Model file for the job. Use its own axes, mm. Give positions to 0.01 mm unless a question says otherwise; leave off trailing zeros. Loops run counter-clockwise (first coordinate to the right, second up) from the corner with the lowest first, then second, coordinate; pieces in that order, holes last. Notation, with made-up numbers: M -19,89.5 L 20,89.5 A33 ccw 20,126.5 Z; hole C 7,55 d8. An arc over 180 degrees is marked long. Answer in a Markdown table with one row per item.
```python
from build123d import *

# Parameters (mm, degrees)
SKETCH1_R           = 4
BOSS_EXTRUDE1_DEPTH = 6
FILLET1_R           = 6
CUT_EXTRUDE1_DEPTH  = 6
FILLET3_R           = 5
SKETCH3_R           = 5.01
CUT_EXTRUDE2_DEPTH  = 10
SKETCH4_W           = 10
SKETCH4_H           = 5
CUT_EXTRUDE3_DEPTH  = 10


with BuildPart() as part:
    # Sketch1 → Boss-Extrude1 (new body)
    with BuildSketch(Plane(origin=(0, 0, 0), x_dir=(1, 0, 0), z_dir=(0, 1, 0))):
        Polygon((277.331893801, -59.723964411), (274.249458289, -59.723964411), (270.793440906, -59.723964411), (225, 0), (95, 0), (95, -35), (0, -35), (0, -135), (95, -135), (95, -170), (225, -170), (270.793440906, -110.276035589), (274.249458289, -110.276035589), (277.331893801, -110.276035589), (323.076052888, -138.788463278), (323.076052888, -148.788463278), (333.076052888, -148.788463278), (368.076052888, -128.788463278), (368.076052888, -41.211536722), (333.076052888, -21.211536722), (323.076052888, -21.211536722), (323.076052888, -31.211536722), align=None)
        with Locations(Location((333.076052888, -138.788463278, 0), (0, 0, 270))):
            Circle(SKETCH1_R, mode=Mode.SUBTRACT)
        with Locations(Location((333.076052888, -31.211536722, 0), (0, 0, 90))):
            Circle(SKETCH1_R, mode=Mode.SUBTRACT)
    extrude(amount=BOSS_EXTRUDE1_DEPTH)

    # Fillet1
    fillet1_edges = [part.edges().sort_by_distance(p)[0] for p in [
        (323.076052888, 3, 31.211536722),
        (323.076052888, 3, 21.211536722),
        (333.076052888, 3, 21.211536722),
        (368.076052888, 3, 41.211536722),
        (368.076052888, 3, 128.788463278),
        (333.076052888, 3, 148.788463278),
        (323.076052888, 3, 148.788463278),
        (323.076052888, 3, 138.788463278),
        (277.331893801, 3, 110.276035589),
        (270.793440906, 3, 110.276035589),
        (225, 3, 170),
        (0, 3, 135),
        (0, 3, 35),
        (225, 3, 0),
        (270.793440906, 3, 59.723964411),
        (277.331893801, 3, 59.723964411),
    ]]
    fillet(fillet1_edges, radius=FILLET1_R)

    # Sketch2 → Cut-Extrude1 (cut)
    with BuildSketch(Plane(origin=(0, 6, 0), x_dir=(1, 0, 0), z_dir=(0, 1, 0))):
        Polygon((261.056483321, -63.459547708), (220.066293487, -10), (220.066293487, -160), (261.056483321, -106.540452292), align=None)
        Polygon((160.709522788, -75.577434726), (208.799641587, -10), (111.200358413, -10), align=None)
        Polygon((111.200358413, -160), (208.799641587, -160), (160.709522788, -94.422565274), align=None)
        Polygon((153.799641587, -85), (105, -18.455034199), (105, -151.544965801), align=None)
        Polygon((52.5, -78.133754394), (87.704614044, -45), (17.295385956, -45), align=None)
        Polygon((17.295385956, -125), (87.704614044, -125), (52.5, -91.866245606), align=None)
        Polygon((45.204614044, -85), (10, -51.866245606), (10, -118.133754394), align=None)
        Polygon((95, -51.866245606), (59.795385956, -85), (95, -118.133754394), align=None)
        Polygon((208.799641587, -139.275270598), (208.799641587, -30.724729402), (167.823301101, -85), align=None)
    extrude(amount=-CUT_EXTRUDE1_DEPTH, mode=Mode.SUBTRACT)

    # Fillet3
    fillet3_edges = [part.edges().sort_by_distance(p)[0] for p in [
        (59.795385956, 3, 85),
        (95, 3, 51.866245606),
        (95, 3, 118.133754394),
        (52.5, 3, 78.133754394),
        (17.295385956, 3, 45),
        (87.704614044, 3, 45),
        (105, 3, 18.455034199),
        (153.799641587, 3, 85),
        (105, 3, 151.544965801),
        (111.200358413, 3, 160),
        (160.709522788, 3, 94.422565274),
        (208.799641587, 3, 160),
        (261.056483321, 3, 63.459547708),
        (261.056483321, 3, 106.540452292),
        (220.066293487, 3, 160),
        (220.066293487, 3, 10),
        (208.799641587, 3, 10),
        (160.709522788, 3, 75.577434726),
        (111.200358413, 3, 10),
        (17.295385956, 3, 125),
        (52.5, 3, 91.866245606),
        (87.704614044, 3, 125),
        (10, 3, 51.866245606),
        (45.204614044, 3, 85),
        (10, 3, 118.133754394),
        (167.823301101, 3, 85),
        (208.799641587, 3, 30.724729402),
        (208.799641587, 3, 139.275270598),
    ]]
    fillet(fillet3_edges, radius=FILLET3_R)

    # Sketch3 → Cut-Extrude2 (cut)
    with BuildSketch(Plane(origin=(0, 6, 0), x_dir=(1, 0, 0), z_dir=(0, 1, 0))):
        with Locations(Location((283.076052888, -100.276035589, 0), (0, 0, 270))):
            Circle(SKETCH3_R)
    extrude(amount=-CUT_EXTRUDE2_DEPTH, mode=Mode.SUBTRACT)

    # Sketch4 → Cut-Extrude3 (cut)
    with BuildSketch(Plane(origin=(0, 6, 0), x_dir=(1, 0, 0), z_dir=(0, 1, 0))):
        with Locations((105, -5)):
            Rectangle(SKETCH4_W, SKETCH4_H)
        with Locations((215.172787049, -5)):
            Rectangle(SKETCH4_W, SKETCH4_H)
        with Locations((215.172787049, -165)):
            Rectangle(SKETCH4_W, SKETCH4_H)
        with Locations((105, -165)):
            Rectangle(SKETCH4_W, SKETCH4_H)
    extrude(amount=-CUT_EXTRUDE3_DEPTH, mode=Mode.SUBTRACT)


solid = part.part
```
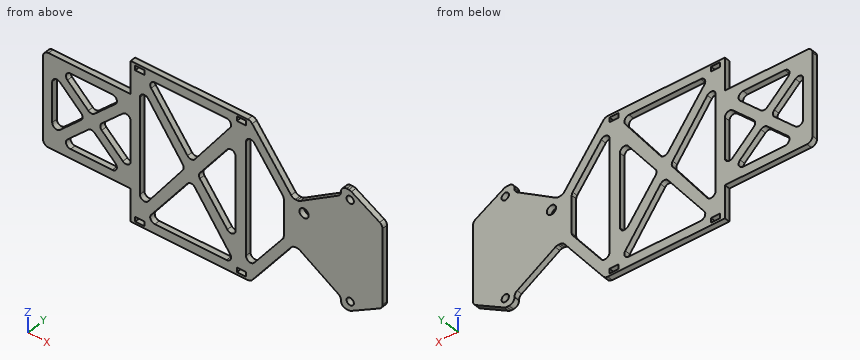
Q1. Saw through at B-B (y = 1.3). Give the number of separate pieces and of enclosed holes in the cut face, and give its area (3 significant figures).
Reported:
| item | result |
|---|---|
| separate pieces | 1 |
| enclosed holes | 16 |
| area | 25,400 mm² |
Q2. Probe probe 1 along X at (y, z) = (4.95, 147) (3 decimals); probe 2 along Z at (x, y) = (199.5, 2.5); probe 3 along X at (y, z) = (1.7, 40.5). List the from-to ranges inside material, lowest first.
Reported:
| item | result |
|---|---|
| probe 1 | 95 to 121.015, 199.266 to 220.378, 230.034 to 242.635, 324.803 to 336.206 |
| probe 2 | 0 to 10.03, 22.68 to 43.04, 126.96 to 147.32, 159.97 to 170 |
| probe 3 | 0.02 to 105, 121.17 to 134.23, 186.43 to 220.07, 243.45 to 256.05, 308.17 to 366.37 |
Q3. Drop flat-ended pins along their axis: pin 1 (1.5 mm diameter, centred on y = 4, z = 164, fed in from +X); pin 2 (1 mm diameter, centred on x = 75.5, y = 3, fed in from +Z); pin 3 (1 mm diameter, centred on x = 309.5, y = 1.5, fed in from +Z); pin 4 (6 mm diameter, centred on x = 283.08, z = 100.28, fed in from -Y). Give the stop position or say it passes through.
Reported:
| item | result |
|---|---|
| pin 1 | x = 230.18 |
| pin 2 | z = 135 |
| pin 3 | z = 130.64 |
| pin 4 | through |
Q4. Saw through at A-A (x = 132.5). Give the cut face in (y, z).
Reported:
| item | result |
|---|---|
| outline | M 0,0 L 6,0 L 6,10 L 0,10 Z; M 0,38.21 L 6,38.21 L 6,55.96 L 0,55.96 Z; M 0,114.04 L 6,114.04 L 6,131.79 L 0,131.79 Z; M 0,160 L 6,160 L 6,170 L 0,170 Z |
